Geometry check sheet. Reference: the model listing, model coordinates, mm. Face numbers are marked on the shaded views. A direction names the side the tool comes from. Coordinates: 2 decimals unless noted, no trailing zeros. Loops run counter-clockwise (first coordinate to the right, second up) from the corner with the lowest first, then second, coordinate; pieces in that order, holes last.
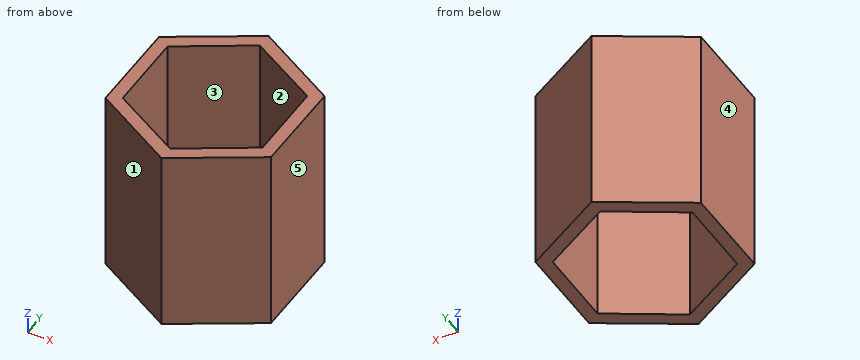
from build123d import *

# Parameters (mm, degrees)
F1_DEPTH = 1
F3_DEPTH = 1
F5_DEPTH = 25.0000003725


with BuildPart() as f1:
    # F0 (on Top) → F1 (new body)
    with BuildSketch(Plane.XY):
        Polygon((10.9985226281, 6.35), (0, 12.7), (-10.9985226281, 6.35), (-10.9985226281, -6.35), (0, -12.7), (10.9985226281, -6.35), align=None)
    extrude(amount=F1_DEPTH)

    # F2 (on Top) → F3 (cut)
    with BuildSketch(Plane.XY):
        Polygon((9.2440988936, 5.389793064), (-0.0456482678, 10.7005210089), (-9.2897471614, 5.310727945), (-9.2440988936, -5.389793064), (0.0456482678, -10.7005210089), (9.2897471614, -5.310727945), align=None)
    extrude(amount=F3_DEPTH, mode=Mode.SUBTRACT)

    # F5 (add): a face of the model
    f5_faces = [f1.faces().sort_by_distance(p)[0] for p in [
        (5.3312561058, 9.2340064434, 1),
    ]]
    extrude(f5_faces, amount=-F5_DEPTH)


solid = f1.part
1) Section check A-A on z = -11. Record the cut outline in (x, y), and give its area (3 significant figures).
Data:
outline: (-11, -6.35) - (0, -12.7) - (11, -6.35) - (11, 6.35) - (0, 12.7) - (-11, 6.35) - close; hole (-9.29, 5.31) - (-9.24, -5.39) - (0.05, -10.7) - (9.29, -5.31) - (9.24, 5.39) - (-0.05, 10.7) - close
area: 122 mm2
2) Depth check by flat-ended pin: pin 1 (12 mm diameter, centred on x = 2, z = -16.5, fed in from +Y); pin 2 (8 mm diameter, centred on x = -7.5, y = 9, fed in from -Z); pin 3 (1 mm diameter, centred on x = -6.5, z = -15, fed in from -Y); pin 4 (8 mm diameter, centred on x = -3.5, z = -9.5, fed in from -Y). Enter the tip coordinate at first touch or a pass-through.
Data:
pin 1: stops at y = 12.7
pin 2: stops at z = -24
pin 3: stops at y = -9.24
pin 4: stops at y = -12.7
3) Section check B-B on x = -8.75. Record the cut outline in (y, z), and give its area (4 significant figures).
Data:
outline: (-7.65, -24) - (-5.67, -24) - (-5.67, 1) - (-7.65, 1) - close; (5.63, -24) - (7.65, -24) - (7.65, 1) - (5.63, 1) - close
area: 100.0 mm2
4) Section check C-C on y = 1.25. Record the cut outline in (x, z), and give its area (3 significant figures).
Data:
outline: (-11, -24) - (-9.27, -24) - (-9.27, 1) - (-11, 1) - close; (9.26, -24) - (11, -24) - (11, 1) - (9.26, 1) - close
area: 86.6 mm2
5) Material ranges on probe 1 along X at (y, z) = (-4.75, -2); probe 2 along X at (y, z) = (10, -9.75); probe 3 along Y at (x, z) = (3.25, -8.25), recorded low to high.
Data:
probe 1: x = -11 to -9.25, 9.29 to 11
probe 2: x = -4.68 to -1.25, 1.18 to 4.68
probe 3: y = -10.82 to -8.83, 8.82 to 10.82
6) Access from +Z, -Z, +X, -X, +Y, -Y to the whole of each face (thin tool, end or side, straight path). Record for the marked faces 1 and 2.
Data:
face 1: +Z, -Z, -X, -Y
face 2: +Z, -Z
7) Mould release check, pull along X, two halves, no side actions. Record for the marked faces 3, 4 and 5: +X half, -X half, draft (parallel to the pull), parting line (faces both ways), or undercut.
Data:
face 3: undercut
face 4: -X half
face 5: +X half
